Can you work these out from the drawing? Everything is in mm from the part's minimum corner. A direction names the side the tool comes from. Coordinates: 2 decimals unless noted, no trailing zeros. Order: outer loops, then holes, each group sorted by start corner. A loop starts at its lowest first (then second) coordinate and runs counter-clockwise, first axis right, second up. Notation, with made-up numbers: M 79,-1 L 105,-1 A20 cw 105,37 Z; hole C 17.5,20.25 d11. An arc over 180 degrees is marked long. Answer as a JSON object with one key per item and string values.
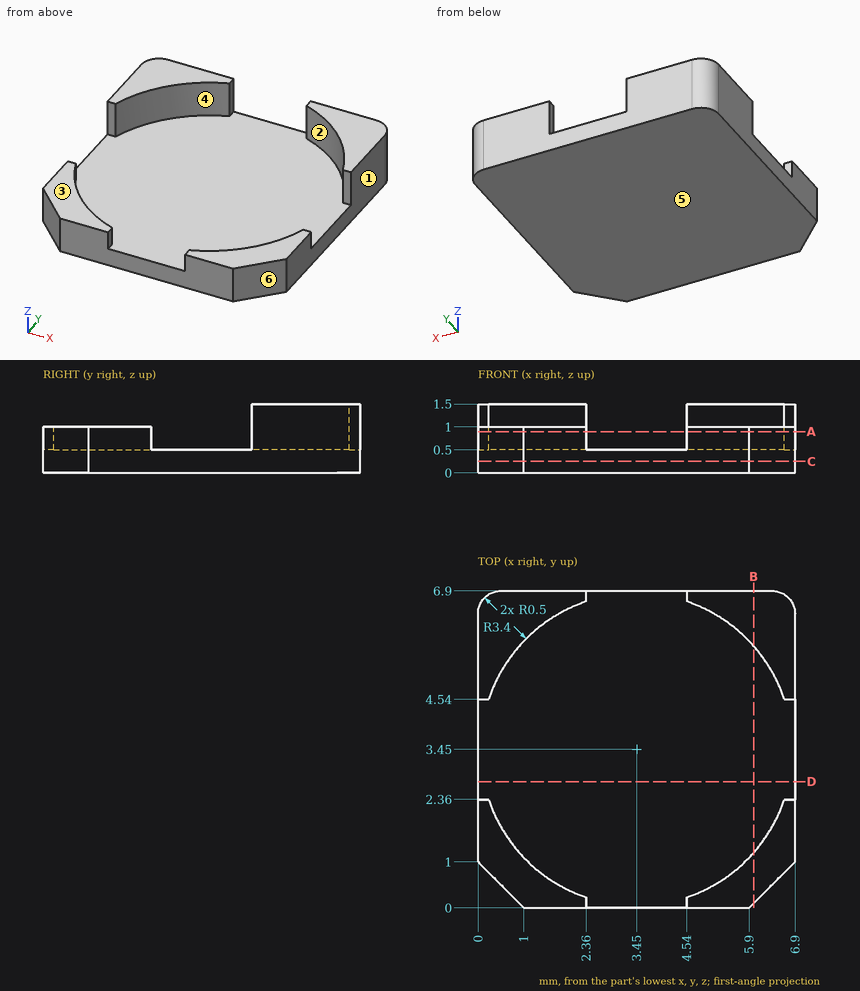
Item 1: I want a section at A-A, the plane z = 0.9. Write out the boundary of the cut face in (x, y).
Answers follow:
{"outline": "M 0,1 L 1,0 L 2.36,0 L 2.36,0.23 A3.4 cw 0.23,2.36 L 0,2.36 Z; M 0,4.54 L 0.23,4.54 A3.4 cw 2.36,6.67 L 2.36,6.9 L 0.5,6.9 A0.5 ccw 0,6.4 Z; M 4.54,0 L 5.9,0 L 6.9,1 L 6.9,2.36 L 6.67,2.36 A3.4 cw 4.54,0.23 Z; M 4.54,6.67 A3.4 cw 6.67,4.54 L 6.9,4.54 L 6.9,6.4 A0.5 ccw 6.4,6.9 L 4.54,6.9 Z"}
Item 2: Please list where these lines run through material, in increasing order: line 1 (Z direction, x = 2.75, y = 2); line 2 (Y direction, x = 0.5, z = 0.75); line 3 (X direction, y = 6.25, z = 1).
Answers follow:
{"line 1": "z = 0 to 0.5", "line 2": "y = 0.5 to 1.76, 5.14 to 6.9", "line 3": "x = 0 to 1.52, 5.38 to 6.9"}
Item 3: If we mould it in two halves opening along Y, with no side actions, what happens to the marked faces 4, 5 and 6? For each: pulls with the +Y half, pulls with the -Y half, needs draft (parallel to the pull), parting line crosses it, or undercut.
Answers follow:
{"face 4": "undercut", "face 5": "needs draft", "face 6": "pulls with the -Y half"}
Item 4: I'm going to push flat-ended pins straight in: pin 1 (4 mm diameter, centred on x = 2, y = 2.5, fed in from +Z); pin 2 (1.5 mm diameter, centred on x = 2, y = 5.5, fed in from +Z). Where does each tip first touch, or does it pass through?
Answers follow:
{"pin 1": "stops at z = 1", "pin 2": "stops at z = 0.5"}
Item 5: I want a section at D-D, the plane y = 2.75. Write out the boundary of the cut face in (x, z).
Answers follow:
{"outline": "M 0,0 L 6.9,0 L 6.9,0.5 L 0,0.5 Z"}
Item 6: Which directions (+Z, -Z, +X, -X, +Y, -Y) give clear straight access to the entire face, cutting with the end or side of a thin tool? Please do the marked faces 1, 2 and 3.
Answers follow:
{"face 1": "+Z, -Z, +X, +Y, -Y", "face 2": "+Z", "face 3": "+Z, +X, -X, -Y"}
Item 7: I want a section at C-C, the plane z = 0.25. Write out the boundary of the cut face in (x, y), plus the area to 3 significant figures.
Answers follow:
{"outline": "M 0,1 L 1,0 L 5.9,0 L 6.9,1 L 6.9,6.4 A0.5 ccw 6.4,6.9 L 0.5,6.9 A0.5 ccw 0,6.4 Z", "area": "46.5 mm^2"}
Item 8: I want a section at B-B, the plane x = 6. Write out the boundary of the cut face in (y, z).
Answers follow:
{"outline": "M 0.1,0 L 6.9,0 L 6.9,1.5 L 5.7,1.5 L 5.7,0.5 L 1.2,0.5 L 1.2,1 L 0.1,1 Z"}
